The listing builds one solid part. Answer for the finished solid, in the listing's coordinates (mm). A direction names the side the tool comes from. Coordinates: 2 decimals unless noted, no trailing zeros. Loops run counter-clockwise (first coordinate to the right, second up) from the corner with the lowest first, then second, coordinate; pieces in that order, holes last. Notation, with made-up numbers: (20.5, 15) - (35.5, 15) arc R19 ccw to (35.5, 32) - close; hole circle Ø7 at (-18.75, 46). An arc over 180 degrees is marked (long way). Write each question's results on one line, items separated by ' | '. Start each with the question number.
(1) Consider line 1 (X direction, y = 24.15, z = -49.8); line 2 (X direction, y = 4.05, z = -10.5); line 3 (X direction, y = 7, z = -48). Determine where each line is inside the solid, lowest interval first. Write a range as from..to.
(2) Find section C-C on z = -107. Determine the outline of the cut face in (x, y).
(3) For faces 1 (the flat face through (84.3, 35.8, -66.6)), 2 (the cylindrical face through (75.57, 39.09, -84.8)), 3 (the flat face through (13.4, 45.8, -42.4)), determine the directions among +Z, -Z, +X, -X, +Y, -Y from which every point of the face is accessible in a straight line to the end or side of a thin tool.
(4) Given pin 1 Ø1.5 at (y, z) = (11, -16) entering from -X; pin 2 Ø7 at (y, z) = (31.5, -85.5) entering from +X; pin 3 Ø1.2 at (x, y) = (74, 37.5) entering from -Z; pin 4 Ø2 at (x, z) = (132.5, -58.5) entering from +Y, each flat-ended and moving along its own axis, determine where each tip first touches the part or whether it passes through.
(5) Find section D-D on x = 107.15. Determine the outline of the cut face in (y, z).
(6) Determine the mould class of faces 4 (the flat face through (9, 37, -40)), 5 (the flat face through (150, 12, -54)), 6 (the cylindrical face through (38.72, 24.01, -51.15)), 7 (the flat face through (74, 12, -110)) for opening direction X: released by +X, released by -X, zero draft, split by the parting line, or undercut.
(7) Find section A-A on y = 16. Determine the outline of the cut face in (x, z).
(8) Find section B-B on x = 39.75. Determine the outline of the cut face in (y, z), then the cut area to 3 significant figures.
from build123d import *

# Parameters (mm, degrees)
SKETCH1_W                = 150
SKETCH1_H                = 110
BOSS_EXTRUDE1_DEPTH      = 25
SKETCH27_R               = 1.9
CONNECTORS_DEPTH         = 4
SKETCH31_W               = 9
SKETCH31_H               = 9
PILLARS_DEPTH            = 15
M3_CLEARANCE_HOLE3_D     = 3.4
M3_CLEARANCE_HOLE3_DEPTH = 5
M3_CLEARANCE_HOLE3_TIP   = 1.021463052
SKETCH33_W               = 5.7
SKETCH33_H               = 2.4
NUT1_DEPTH               = 10
SKETCH34_W               = 5.6
SKETCH34_H               = 2.4
NUT2_DEPTH               = 10
SKETCH37_W               = 5.6
SKETCH37_H               = 2.4
NUT5_DEPTH               = 10
SKETCH38_W               = 5.6
SKETCH38_H               = 2.4
NUT6_DEPTH               = 10
SKETCH10_W               = 85.5
SKETCH10_H               = 78
BATTERY_HOLDER_DEPTH     = 23
SKETCH39_W               = 7
SKETCH39_H               = 60
DIVIDER_DEPTH            = 10
M3_CLEARANCE_HOLE4_D     = 3.4
M3_CLEARANCE_HOLE4_DEPTH = 5
M3_CLEARANCE_HOLE4_TIP   = 1.021463052
SKETCH41_W               = 10
SKETCH41_H               = 5
BATTERY_WIRE_DEPTH       = 2
SKETCH42_R               = 2
CONNECTOR_BOTTOM_DEPTH   = 5
SKETCH43_W               = 54
SKETCH43_H               = 9
PCB_REST_DEPTH           = 15
SKETCH44_W               = 5.6
SKETCH44_H               = 2.4
NUT3_DEPTH               = 10
SKETCH45_W               = 5.6
SKETCH45_H               = 2.4
NUT4_DEPTH               = 10
SKETCH46_W               = 5.6
SKETCH46_H               = 2.4
NUT7_DEPTH               = 10
SKETCH48_W               = 9
SKETCH48_H               = 9
PCBINPUT_PILLARS_DEPTH   = 25
NUT8_REACH               = 187.691
SKETCH49_W               = 5.6
SKETCH49_H               = 2.4
NUT9_REACH               = 187.691
SKETCH50_W               = 5.6
SKETCH50_H               = 2.4
M3_CLEARANCE_HOLE5_D     = 3.4
M3_CLEARANCE_HOLE5_DEPTH = 5
M3_CLEARANCE_HOLE5_TIP   = 1.021463052


with BuildPart() as part:
    # Sketch1 → Boss-Extrude1 (new body)
    with BuildSketch(Plane(origin=(0, 0, 0), x_dir=(1, 0, 0), z_dir=(0, 1, 0))):
        with Locations((75, 55)):
            Rectangle(SKETCH1_W, SKETCH1_H)
    extrude(amount=BOSS_EXTRUDE1_DEPTH)

    # Sketch27 → Connectors (add)
    with BuildSketch(Plane(origin=(0, 25, 0), x_dir=(1, 0, 0), z_dir=(0, 1, 0))):
        with Locations(Location((3, 107, 0), (0, 0, 90))):
            Circle(SKETCH27_R)
        with Locations(Location((75, 107, 0), (0, 0, 90))):
            Circle(SKETCH27_R)
        with Locations(Location((147, 107, 0), (0, 0, 90))):
            Circle(SKETCH27_R)
        with Locations(Location((147, 55, 0), (0, 0, 90))):
            Circle(SKETCH27_R)
        with Locations(Location((147, 3, 0), (0, 0, 90))):
            Circle(SKETCH27_R)
        with Locations(Location((75, 3, 0), (0, 0, 90))):
            Circle(SKETCH27_R)
        with Locations(Location((3, 3, 0), (0, 0, 90))):
            Circle(SKETCH27_R)
        with Locations(Location((3, 55, 0), (0, 0, 90))):
            Circle(SKETCH27_R)
    extrude(amount=CONNECTORS_DEPTH)

    # Sketch31 → Pillars (add)
    with BuildSketch(Plane(origin=(0, 25, 0), x_dir=(1, 0, 0), z_dir=(0, 1, 0))):
        with Locations((122.5, 86.5)):
            Rectangle(SKETCH31_W, SKETCH31_H)
        with Locations((25.25, 15)):
            Rectangle(SKETCH31_W, SKETCH31_H)
        with Locations((62.75, 14.5)):
            Rectangle(SKETCH31_W, SKETCH31_H)
        with Locations((114.75, 41)):
            Rectangle(SKETCH31_W, SKETCH31_H)
        with Locations((84.25, 68.5)):
            Rectangle(SKETCH31_W, SKETCH31_H)
        with Locations((75.5, 86.5)):
            Rectangle(SKETCH31_W, SKETCH31_H)
        with Locations((27.5, 86.5)):
            Rectangle(SKETCH31_W, SKETCH31_H)
    extrude(amount=PILLARS_DEPTH)

    # M3 Clearance Hole3
    with Locations(Plane(origin=(84.25, 40, -68.5), x_dir=(0, 0, 1), z_dir=(0, 1, 0))):
        with Locations((0, 0), (27.5, 30.5), (54, -21.5), (53.5, -59), (-18, -56.75), (-18, -8.75), (-18, 38.25)):
            Hole(M3_CLEARANCE_HOLE3_D / 2, depth=M3_CLEARANCE_HOLE3_DEPTH)
            with Locations((0, 0, -(M3_CLEARANCE_HOLE3_DEPTH + M3_CLEARANCE_HOLE3_TIP / 2))):  # 118° drill point
                Cone(0, M3_CLEARANCE_HOLE3_D / 2, M3_CLEARANCE_HOLE3_TIP, mode=Mode.SUBTRACT)

    # Sketch33 → Nut1 (cut)
    with BuildSketch(Plane(origin=(119.25, 0, 0), x_dir=(0, 0, -1), z_dir=(1, 0, 0))):
        with Locations((41, 37)):
            Rectangle(SKETCH33_W, SKETCH33_H)
    extrude(amount=-NUT1_DEPTH, mode=Mode.SUBTRACT)

    # Sketch34 → Nut2 (cut)
    with BuildSketch(Plane(origin=(88.75, 0, 0), x_dir=(0, 0, -1), z_dir=(1, 0, 0))):
        with Locations((68.5, 37)):
            Rectangle(SKETCH34_W, SKETCH34_H)
    extrude(amount=-NUT2_DEPTH, mode=Mode.SUBTRACT)

    # Sketch37 → Nut5 (cut)
    with BuildSketch(Plane(origin=(67.25, 0, 0), x_dir=(0, 0, -1), z_dir=(1, 0, 0))):
        with Locations((14.5, 37)):
            Rectangle(SKETCH37_W, SKETCH37_H)
    extrude(amount=-NUT5_DEPTH, mode=Mode.SUBTRACT)

    # Sketch38 → Nut6 (cut)
    with BuildSketch(Plane(origin=(29.75, 0, 0), x_dir=(0, 0, -1), z_dir=(1, 0, 0))):
        with Locations((15, 37)):
            Rectangle(SKETCH38_W, SKETCH38_H)
    extrude(amount=-NUT6_DEPTH, mode=Mode.SUBTRACT)

    # Sketch10 → Battery holder (cut)
    with BuildSketch(Plane.XZ):
        with Locations((75, -51)):
            Rectangle(SKETCH10_W, SKETCH10_H)
    extrude(amount=-BATTERY_HOLDER_DEPTH, mode=Mode.SUBTRACT)

    # Sketch39 → Divider (add)
    with BuildSketch(Plane.XZ.offset(-23)):
        with Locations((73.25, -46)):
            Rectangle(SKETCH39_W, SKETCH39_H)
    extrude(amount=DIVIDER_DEPTH)

    # M3 Clearance Hole4
    with Locations(Plane(origin=(107.15, 23, -49.8), x_dir=(0, 0, -1), z_dir=(0, -1, 0))):
        with Locations((0, 0), (0, -19.4), (0, -48), (0, -67.4)):
            Hole(M3_CLEARANCE_HOLE4_D / 2, depth=M3_CLEARANCE_HOLE4_DEPTH)
            with Locations((0, 0, -(M3_CLEARANCE_HOLE4_DEPTH + M3_CLEARANCE_HOLE4_TIP / 2))):  # 118° drill point
                Cone(0, M3_CLEARANCE_HOLE4_D / 2, M3_CLEARANCE_HOLE4_TIP, mode=Mode.SUBTRACT)

    # Sketch41 → Battery wire (cut)
    with BuildSketch(Plane.XZ.offset(-23)):
        with Locations((97.25, -85.5)):
            Rectangle(SKETCH41_W, SKETCH41_H)
        with Locations((52.75, -85.5)):
            Rectangle(SKETCH41_W, SKETCH41_H)
    extrude(amount=-BATTERY_WIRE_DEPTH, mode=Mode.SUBTRACT)

    # Sketch42 → Connector bottom (cut)
    with BuildSketch(Plane.XZ):
        with Locations(Location((119.25, -10.5, 0), (0, 0, 270))):
            Circle(SKETCH42_R)
        with Locations(Location((30.75, -10.5, 0), (0, 0, 270))):
            Circle(SKETCH42_R)
        with Locations(Location((30.75, -91.5, 0), (0, 0, 270))):
            Circle(SKETCH42_R)
        with Locations(Location((119.25, -91.5, 0), (0, 0, 270))):
            Circle(SKETCH42_R)
    extrude(amount=-CONNECTOR_BOTTOM_DEPTH, mode=Mode.SUBTRACT)

    # Sketch43 → PCB rest (add)
    with BuildSketch(Plane(origin=(0, 25, 0), x_dir=(1, 0, 0), z_dir=(0, 1, 0))):
        with Locations((47.25, 67)):
            Rectangle(SKETCH43_W, SKETCH43_H)
    extrude(amount=PCB_REST_DEPTH)

    # Sketch44 → Nut3 (cut)
    with BuildSketch(Plane(origin=(127, 0, 0), x_dir=(0, 0, -1), z_dir=(1, 0, 0))):
        with Locations((86.5, 37)):
            Rectangle(SKETCH44_W, SKETCH44_H)
    extrude(amount=-NUT3_DEPTH, mode=Mode.SUBTRACT)

    # Sketch45 → Nut4 (cut)
    with BuildSketch(Plane(origin=(80, 0, 0), x_dir=(0, 0, -1), z_dir=(1, 0, 0))):
        with Locations((86.5, 37)):
            Rectangle(SKETCH45_W, SKETCH45_H)
    extrude(amount=-NUT4_DEPTH, mode=Mode.SUBTRACT)

    # Sketch46 → Nut7 (cut)
    with BuildSketch(Plane(origin=(32, 0, 0), x_dir=(0, 0, -1), z_dir=(1, 0, 0))):
        with Locations((86.5, 37)):
            Rectangle(SKETCH46_W, SKETCH46_H)
    extrude(amount=-NUT7_DEPTH, mode=Mode.SUBTRACT)

    # Sketch48 → PCBInput pillars (add)
    with BuildSketch(Plane(origin=(0, 25, 0), x_dir=(1, 0, 0), z_dir=(0, 1, 0))):
        with Locations((13.5, 40.5)):
            Rectangle(SKETCH48_W, SKETCH48_H)
        with Locations((13.5, 21.5)):
            Rectangle(SKETCH48_W, SKETCH48_H)
    extrude(amount=PCBINPUT_PILLARS_DEPTH)

    # Sketch49 → Nut8 (cut, up to next)
    with BuildSketch(Plane.ZY.offset(-9), mode=Mode.PRIVATE) as nut8_sk1:
        with Locations((-21.5, 47)):
            Rectangle(SKETCH49_W, SKETCH49_H)
    nut8_tool1 = extrude(nut8_sk1.sketch, amount=-NUT8_REACH, mode=Mode.PRIVATE) & part.part
    add(nut8_tool1.solids().sort_by_distance((9, 47, -21.5))[0], mode=Mode.SUBTRACT)

    # Sketch50 → Nut9 (cut, up to next)
    with BuildSketch(Plane.ZY.offset(-9), mode=Mode.PRIVATE) as nut9_sk1:
        with Locations((-40.5, 47)):
            Rectangle(SKETCH50_W, SKETCH50_H)
    nut9_tool1 = extrude(nut9_sk1.sketch, amount=-NUT9_REACH, mode=Mode.PRIVATE) & part.part
    add(nut9_tool1.solids().sort_by_distance((9, 47, -40.5))[0], mode=Mode.SUBTRACT)

    # M3 Clearance Hole5
    with Locations(Plane(origin=(13.5, 50, -40.5), x_dir=(0, 0, 1), z_dir=(0, 1, 0))):
        with Locations((0, 0), (19, 0)):
            Hole(M3_CLEARANCE_HOLE5_D / 2, depth=M3_CLEARANCE_HOLE5_DEPTH)
            with Locations((0, 0, -(M3_CLEARANCE_HOLE5_DEPTH + M3_CLEARANCE_HOLE5_TIP / 2))):  # 118° drill point
                Cone(0, M3_CLEARANCE_HOLE5_D / 2, M3_CLEARANCE_HOLE5_TIP, mode=Mode.SUBTRACT)


solid = part.part
Values:
1) line 1: x = 0..38.05, 41.45..57.45, 60.85..86.05, 89.45..105.45, 108.85..150 | line 2: x = 0..28.75, 32.75..117.25, 121.25..150 | line 3: x = 0..32.25, 117.75..150
2) outline: (0, 0) - (150, 0) - (150, 25) - (148.9, 25) - (148.9, 29) - (145.1, 29) - (145.1, 25) - (76.9, 25) - (76.9, 29) - (73.1, 29) - (73.1, 25) - (4.9, 25) - (4.9, 29) - (1.1, 29) - (1.1, 25) - (0, 25) - close
3) face 1: +X | face 2: +Y | face 3: +X, -X
4) pin 1: stops at x = 0 | pin 2: stops at x = 127 | pin 3: stops at z = -91 | pin 4: stops at y = 25
5) outline: (0, -110) - (25, -110) - (25, -51.5) - (23, -51.5) - (23, -90) - (0, -90) - close; (0, -12) - (23, -12) - (23, -48.1) - (25, -48.1) - (25, 0) - (0, 0) - close
6) face 4: released by -X | face 5: released by +X | face 6: undercut | face 7: zero draft
7) outline: (0, -110) - (150, -110) - (150, 0) - (0, 0) - close; (69.75, -76) - (76.75, -76) - (76.75, -16) - (69.75, -16) - close; hole (32.25, -90) - (117.75, -90) - (117.75, -12) - (32.25, -12) - close
8) outline: (0, -110) - (25, -110) - (25, -71.5) - (40, -71.5) - (40, -62.5) - (25, -62.5) - (25, -51.5) - (23, -51.5) - (23, -90) - (0, -90) - close; (0, -12) - (23, -12) - (23, -48.1) - (25, -48.1) - (25, 0) - (0, 0) - close | area: 1,080 mm²
